```python
from build123d import *

# Parameters (mm, degrees)
ESTRUSIONE_ESTRUSIONE1_DEPTH = 30
RACCORDO1_R                  = 15
RACCORDO2_R                  = 160


with BuildPart() as part:
    # Schizzo1 → Estrusione-Estrusione1 (new body)
    with BuildSketch(Plane.XY):
        with BuildLine():
            Line((-46.448079544, 63.011055337), (-33.755592428, 70.09420993))
            Line((-33.755592428, 70.09420993), (-20.304122895, 75.601321294))
            ThreePointArc((-20.304122895, 75.601321294), (-13.252536333, 75.502654626), (-8.436946182, 70.35049977))
            Line((-8.436946182, 70.35049977), (-8, 69.15))
            ThreePointArc((-8, 69.15), (0, 61.15), (8, 69.15))
            Line((8, 69.15), (8.436946182, 70.35049977))
            ThreePointArc((8.436946182, 70.35049977), (13.252536333, 75.502654626), (20.304122895, 75.601321294))
            Line((20.304122895, 75.601321294), (33.755592428, 70.09420993))
            Line((33.755592428, 70.09420993), (46.448079544, 63.011055337))
            ThreePointArc((46.448079544, 63.011055337), (50.767531144, 57.4363853), (49.741885624, 50.459089304))
            Line((49.741885624, 50.459089304), (49.075728598, 49.368971658))
            ThreePointArc((49.075728598, 49.368971658), (47.808995153, 38.126401384), (59.051565428, 36.859667939))
            Line((59.051565428, 36.859667939), (60.262585431, 37.266549021))
            ThreePointArc((60.262585431, 37.266549021), (67.293173649, 36.713885045), (71.766906665, 31.262250331))
            Line((71.766906665, 31.262250331), (75.848127696, 17.311840191))
            Line((75.848127696, 17.311840191), (78.223930717, 2.97217952))
            ThreePointArc((78.223930717, 2.97217952), (76.558612201, -3.880653646), (70.464063006, -7.429044586))
            Line((70.464063006, -7.429044586), (69.196432599, -7.587899286))
            ThreePointArc((69.196432599, -7.587899286), (59.61684183, -13.607155111), (65.636097656, -23.186745881))
            Line((65.636097656, -23.186745881), (66.709268717, -23.87987324))
            ThreePointArc((66.709268717, -23.87987324), (70.660678677, -29.721188801), (69.187745938, -36.617932765))
            Line((69.187745938, -36.617932765), (60.82547579, -48.506698308))
            Line((60.82547579, -48.506698308), (51.095566584, -59.304808098))
            ThreePointArc((51.095566584, -59.304808098), (44.699496759, -62.275481245), (38.12536374, -59.722956378))
            Line((38.12536374, -59.722956378), (37.210811503, -58.830927303))
            ThreePointArc((37.210811503, -58.830927303), (26.531990647, -55.094246272), (22.795309617, -65.773067128))
            Line((22.795309617, -65.773067128), (22.922512038, -67.04426389))
            ThreePointArc((22.922512038, -67.04426389), (20.819251446, -73.775601279), (14.508801347, -76.92406562))
            Line((14.508801347, -76.92406562), (0, -77.798703626))
            Line((0, -77.798703626), (-14.508801347, -76.92406562))
            ThreePointArc((-14.508801347, -76.92406562), (-20.819251446, -73.775601279), (-22.922512038, -67.04426389))
            Line((-22.922512038, -67.04426389), (-22.795309617, -65.773067128))
            ThreePointArc((-22.795309617, -65.773067128), (-26.531990647, -55.094246272), (-37.210811503, -58.830927303))
            Line((-37.210811503, -58.830927303), (-38.12536374, -59.722956378))
            ThreePointArc((-38.12536374, -59.722956378), (-44.699496759, -62.275481245), (-51.095566584, -59.304808098))
            Line((-51.095566584, -59.304808098), (-60.82547579, -48.506698308))
            Line((-60.82547579, -48.506698308), (-69.187745938, -36.617932765))
            ThreePointArc((-69.187745938, -36.617932765), (-70.660678677, -29.721188801), (-66.709268717, -23.87987324))
            Line((-66.709268717, -23.87987324), (-65.636097656, -23.186745881))
            ThreePointArc((-65.636097656, -23.186745881), (-59.61684183, -13.607155111), (-69.196432599, -7.587899286))
            Line((-69.196432599, -7.587899286), (-70.464063006, -7.429044586))
            ThreePointArc((-70.464063006, -7.429044586), (-76.558612201, -3.880653646), (-78.223930717, 2.97217952))
            Line((-78.223930717, 2.97217952), (-75.848127696, 17.311840191))
            Line((-75.848127696, 17.311840191), (-71.766906665, 31.262250331))
            ThreePointArc((-71.766906665, 31.262250331), (-67.293173649, 36.713885045), (-60.262585431, 37.266549021))
            Line((-60.262585431, 37.266549021), (-59.051565428, 36.859667939))
            ThreePointArc((-59.051565428, 36.859667939), (-47.808995153, 38.126401384), (-49.075728598, 49.368971658))
            Line((-49.075728598, 49.368971658), (-49.741885624, 50.459089304))
            ThreePointArc((-49.741885624, 50.459089304), (-50.767531144, 57.4363853), (-46.448079544, 63.011055337))
        make_face()
    extrude(amount=ESTRUSIONE_ESTRUSIONE1_DEPTH)

    # Raccordo1
    # the kernel refuses this fillet: 15 mm, written as the material it takes off along each edge
    with BuildSketch(Plane(origin=(8, 69.15, -3.193862928), x_dir=(-0.06981955968385771, -0.9975596368566404, 0), z_dir=(0, 0, 1)), Plane(origin=(-49.075728598, 49.368971658, -3.193862928), x_dir=(0.7363917463007478, -0.6765553901789085, 0), z_dir=(0, 0, 1)), Plane(origin=(-69.196432599, -7.587899286, -3.193862928), x_dir=(0.9880850476667732, 0.15390886451842375, 0), z_dir=(0, 0, 1)), Plane(origin=(-37.210811503, -58.830927303, -3.193862928), x_dir=(0.49573015487791666, 0.8684766050647056, 0), z_dir=(0, 0, 1)), Plane(origin=(22.795309617, -65.773067128, -3.193862928), x_dir=(-0.3699196555863113, 0.9290637483030455, 0), z_dir=(0, 0, 1)), Plane(origin=(65.636097656, -23.186745881, -3.193862928), x_dir=(-0.9570124204082326, 0.2900469396224969, 0), z_dir=(0, 0, 1)), Plane(origin=(59.051565428, 36.859667939, -3.193862928), x_dir=(-0.8234553131670451, -0.5673811304731269, 0), z_dir=(0, 0, 1))) as raccordo1_piece_1:
        with BuildLine():
            CenterArc((2.16440635, 14.963394553), RACCORDO1_R, 256.928571472, 9.067805135)
            Line((-1.228077505, 0.35206151), (-1.295927182, 0.059834849))
            ThreePointArc((-1.295927182, 0.059834849), (-0.696711722, -0.112352983), (-0.082672969, -0.288383738))
            Line((-0.082672969, -0.288383738), (0.020945868, -0.299267891))
            ThreePointArc((0.020945868, -0.299267891), (0.558556477, -0.280477095), (1.096167087, -0.299267891))
            Line((1.096167087, -0.299267891), (1.117112955, 0))
        make_face()
    extrude(amount=36.387725855, mode=Mode.SUBTRACT)
    with BuildSketch(Plane(origin=(-59.051565428, 36.859667939, -3.193862928), x_dir=(-0.9479273461671341, 0.31848665025167716, 0), z_dir=(0, 0, 1)), Plane(origin=(-65.636097656, -23.186745881, -3.193862928), x_dir=(-0.840025923150775, -0.542546263865754, 0), z_dir=(0, 0, 1)), Plane(origin=(-22.795309617, -65.773067128, -3.193862928), x_dir=(-0.09956784659581282, -0.9950307753654017, 0), z_dir=(0, 0, 1)), Plane(origin=(37.210811503, -58.830927303, -3.193862928), x_dir=(0.7158668492597241, -0.698236818086067, 0), z_dir=(0, 0, 1)), Plane(origin=(69.196432599, -7.587899286, -3.193862928), x_dir=(0.9922392066001717, 0.12434370464748737, 0), z_dir=(0, 0, 1)), Plane(origin=(49.075728598, 49.368971658, -3.193862928), x_dir=(0.5214352033794836, 0.8532908816321646, 0), z_dir=(0, 0, 1)), Plane(origin=(-8, 69.15, -3.193862928), x_dir=(-0.3420201433256726, 0.9396926207859071, 0), z_dir=(0, 0, 1))) as raccordo1_piece_2:
        with BuildLine():
            CenterArc((2.042962228, 14.980458495), RACCORDO1_R, 258.007246785, 9.067805135)
            Line((-1.073857364, 0.307850151), (-1.136193756, 0.014397984))
            ThreePointArc((-1.136193756, 0.014397984), (-0.614221596, -0.115691701), (-0.102606043, -0.281907786))
            Line((-0.102606043, -0.281907786), (0, -0.3))
            ThreePointArc((0, -0.3), (0.638772586, -0.3), (1.26223683, -0.29960917))
            Line((1.26223683, -0.29960917), (1.277545171, 0))
        make_face()
    extrude(amount=36.387725855, mode=Mode.SUBTRACT)

    # Raccordo2
    raccordo2_edges = [part.edges().sort_by_distance(p)[0] for p in [
        (-33.755592428, 70.09420993, 15),
        (33.755592428, 70.09420993, 15),
        (75.848127696, 17.311840191, 15),
        (60.82547579, -48.506698308, 15),
        (0, -77.798703626, 15),
        (-60.82547579, -48.506698308, 15),
        (-75.848127696, 17.311840191, 15),
    ]]
    fillet(raccordo2_edges, radius=RACCORDO2_R)


solid = part.part
```
Here's how the part is built. I have some questions about the finished solid (model axes, mm). Give positions to 0.01 mm unless a question says otherwise; leave off trailing zeros. Loops run counter-clockwise (first coordinate to the right, second up) from the corner with the lowest first, then second, coordinate; pieces in that order, holes last. Notation, with made-up numbers: M 12.5,21.5 L 63.5,21.5 A13 ccw 63.5,35.5 Z; hole C 71.25,23 d5. An arc over 180 degrees is marked long. Return JSON: item names as keys, results as strings.
Item 1: Imagine slicing it at B-B on y = -30.5. List the corners of the cut face in (x, z) for me.
A:
{"outline": "M -70.78,0 L 70.78,0 L 70.78,30 L -70.78,30 Z"}
Item 2: Thinking about a two-plate mould opening in Y: for faces 1 (the cylindrical face through (-50.793, 57.338, 14.79)), 2 (the cylindrical face through (44.8, -62.27, 14.79)), 3 (the flat face through (44.28, 64.22, 14.79)), 4 (the cylindrical face through (-47.91, 38, 14.79)), which applies, released by +Y, released by -Y, zero draft, split by the parting line, or undercut?
A:
{"face 1": "undercut", "face 2": "released by -Y", "face 3": "released by +Y", "face 4": "undercut"}
Item 3: I'm going to push flat-ended pins straight in: pin 1 Ø3 at (x, z) = (-58.5, 22) entering from +Y; pin 2 Ø10 at (x, y) = (34.5, 46.5) entering from -Z; pin 3 Ø10 at (x, z) = (-39, 21) entering from -Y; pin 4 Ø6 at (x, z) = (-58.5, 6.5) entering from +Y. Where does each tip first touch, or does it pass through?
A:
{"pin 1": "stops at y = 37.16", "pin 2": "stops at z = 0", "pin 3": "stops at y = -62.27", "pin 4": "stops at y = 37.59"}
Item 4: Imagine slicing it at A-A on x = 5. List the corners of the cut face in (y, z) for me (3 decimals), then the cut area to 3 significant figures.
A:
{"outline": "M -77.43,0 L 62.905,0 L 62.905,30 L -77.43,30 Z", "area": "4,210 mm^2"}
Item 5: Please list where these lines run through material, in increasing order: line 1 (X direction, y = -55, z = 3.25); line 2 (X direction, y = -58.5, z = 23); line 3 (X direction, y = 62.5, z = 6).
A:
{"line 1": "x = -54.97 to -33.27, -26.73 to 26.73, 33.27 to 54.97", "line 2": "x = -51.82 to -37.11, -22.96 to 22.96, 37.11 to 51.82", "line 3": "x = -47.26 to -4.45, 4.45 to 47.26"}
